The model under review builds one solid part; all positions refer to its coordinate system, in mm. Face numbers are marked on the shaded views. Give positions to 0.01 mm unless a question says otherwise; leave off trailing zeros. Loops run counter-clockwise (first coordinate to the right, second up) from the corner with the lowest first, then second, coordinate; pieces in that order, holes last. Notation, with made-up numbers: (8.5, -25.5) - (47.5, -25.5) arc R31 cw to (47.5, -0.5) - close; hole circle Ø1 at (-2.75, 47). An arc over 180 degrees is marked (long way). Answer as a JSON object with one key per item and string values.
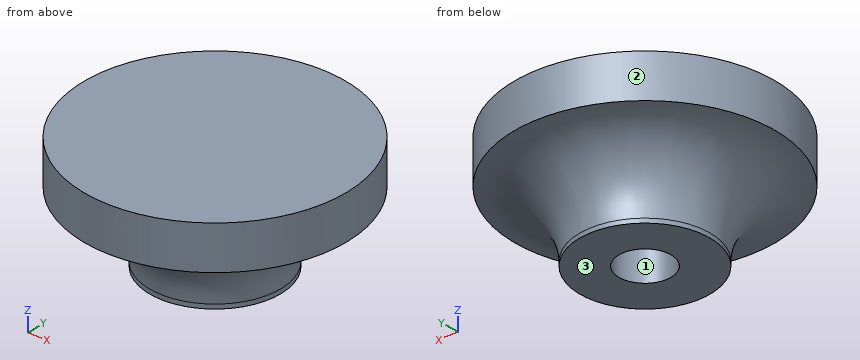
from build123d import *

# Parameters (mm, degrees)
SKETCH129_R             = 15
PAD067_DEPTH            = 5
SKETCH130_R             = 7.5
SKETCH130_R_2           = 3
PAD068_DEPTH            = 8
FILLET001_R             = 7.49999
BODY018_PLACEMENT_ANGLE = 90


with BuildPart() as part:
    # Sketch129 → Pad067 (new body)
    with BuildSketch(Plane.YZ):
        Circle(SKETCH129_R)
    extrude(amount=PAD067_DEPTH)

    # Sketch130 (on Face3 of Pad067) → Pad068 (join)
    with BuildSketch(Plane.YZ.offset(5)):
        Circle(SKETCH130_R)
        Circle(SKETCH130_R_2, mode=Mode.SUBTRACT)
    extrude(amount=PAD068_DEPTH)

    # Fillet001
    fillet001_edges = [part.edges().sort_by_distance(p)[0] for p in [
        (5, -7.5, 0),
    ]]
    fillet(fillet001_edges, radius=FILLET001_R)


with BuildPart() as part_1:
    # Body018 placement: moved
    add(part.part.moved(Location((-100, -121.8, -33.01))).rotate(Axis((-100, -121.8, -33.01), (0, 1, 0)), BODY018_PLACEMENT_ANGLE))


solid = part_1.part
Q1. The part is to be moulded in two halves that separate along X. For the marked faces 1, 2 and 3, say which applies: +X half, -X half, draft (parallel to the pull), parting line (faces both ways), or undercut.
Results:
{"face 1": "undercut", "face 2": "parting line", "face 3": "draft"}
Q2. To check wall thickness, follow probe 1 along X at (y, z) = (-121.8, -40.25); probe 2 along X at (y, z) = (-121.8, -42.75); probe 3 along Z at (x, y) = (-102.5, -121). State the ranges of each line that lie inside material, in increasing order. Write a range as [from, to].
Results:
{"probe 1": "x = [-109.65, -103], [-97, -90.35]", "probe 2": "x = [-108.03, -103], [-97, -91.97]", "probe 3": "z = [-38.01, -33.01]"}
Q3. Consider section C-C, the plane z = -35. State the section outline as (x, y) points, plus the area to 3 significant figures.
Results:
{"outline": "circle Ø30 at (-100, -121.8)", "area": "707 mm^2"}
Q4. Clearance check with flat-ended pins moving along their axes: pin 1 Ø4 at (y, z) = (-123.5, -36) entering from +X; pin 2 Ø5 at (y, z) = (-113, -36.5) entering from +X; pin 3 Ø1 at (x, y) = (-89, -113.5) entering from -Z; pin 4 Ø1 at (y, z) = (-119, -35) entering from +X. State where each tip first meets the part, or that it passes through.
Results:
{"pin 1": "stops at x = -85", "pin 2": "stops at x = -86.39", "pin 3": "stops at z = -38.21", "pin 4": "stops at x = -85.18"}
Q5. Consider section D-D, the plane z = -39.75. State the section outline as (x, y) points.
Results:
{"outline": "circle Ø20.39 at (-100, -121.8); hole circle Ø6 at (-100, -121.8)"}
